Autodesk Fusion 360 part; units mm, degrees
sketch "Esquisse1" plane through (0, 0, 0) normal (0, 0, 1) x (1, 0, 0)
  line L0 (0, 0) -> (58, 0)
  line L1 (58, 0) -> (58, 8)
  line L2 (58, 8) -> (0, 8)
  line L3 (0, 8) -> (0, 0)
  dimension "d1" = 58
  dimension "d2" = 8
extrude "Extrusion1" add sketch "Esquisse1" along normal blind 2
sketch "Esquisse2" plane through (0, 0, 2) normal (0, 0, 1) x (-1, 0, 0)
  line L0 (0, -8) -> (0, 0)
  line L1 (0, 0) -> (-58, 0)
  line L2 (-58, 0) -> (-58, -8)
  line L3 (-58, -8) -> (0, -8)
  line L4 (0, -8) -> (-58, -8)
  line L5 (-58, -8) -> (-58, -6)
  line L6 (-58, -6) -> (0, -6)
  line L7 (0, -6) -> (0, -8)
  dimension "d5" = 2
extrude "Extrusion2" add sketch "Esquisse2" along normal blind 2 contours L0 L2 L3 L4 L5 L6 L7
Design review of the part built by this model. Coordinates are the model's own, in mm. A direction names the side the tool comes from. Coordinates: 2 decimals unless noted, no trailing zeros. Loops run counter-clockwise (first coordinate to the right, second up) from the corner with the lowest first, then second, coordinate; pieces in that order, holes last.
Item 1: Wall thickness on L1, parallel to Z at x = 43, y = 0.75; L2, parallel to Y at x = 27.5, z = 2.8: over which ranges is each line inside the solid? List them lowest first.
Completed:
L1: z = 0 to 2
L2: y = 6 to 8
Item 2: Add section B-B (z = 3.25). Write out the cut boundary in (x, y), and give its area (3 significant figures).
Completed:
outline: (0, 6) - (58, 6) - (58, 8) - (0, 8) - close
area: 116 mm2
Item 3: For faces 1 (the flat face through (29, 6, 3)), 2 (the flat face through (0, 4.9, 1.5)), list the 3-axis set-ups (+Z, -Z, +X, -X, +Y, -Y) from which the entire face can be reached by the end or side of a thin tool; tool diameter is ignored.
Completed:
face 1: +Z, +X, -X, -Y
face 2: +Z, -Z, -X, +Y, -Y
Item 4: Add section C-C (y = 4). Write out the cut boundary in (x, z), and give its area (3 significant figures).
Completed:
outline: (0, 0) - (58, 0) - (58, 2) - (0, 2) - close
area: 116 mm2
Item 5: Add section A-A (x = 54). Write out the cut boundary in (y, z).
Completed:
outline: (0, 0) - (8, 0) - (8, 4) - (6, 4) - (6, 2) - (0, 2) - close
Item 6: Clearance check with a flat-ended pin moving along its axis: pin 1 (0.6 mm diameter, centred on x = 38, z = 2.5, fed in from -Y). State where the tip first meets the part, or that it passes through.
Completed:
pin 1: stops at y = 6
